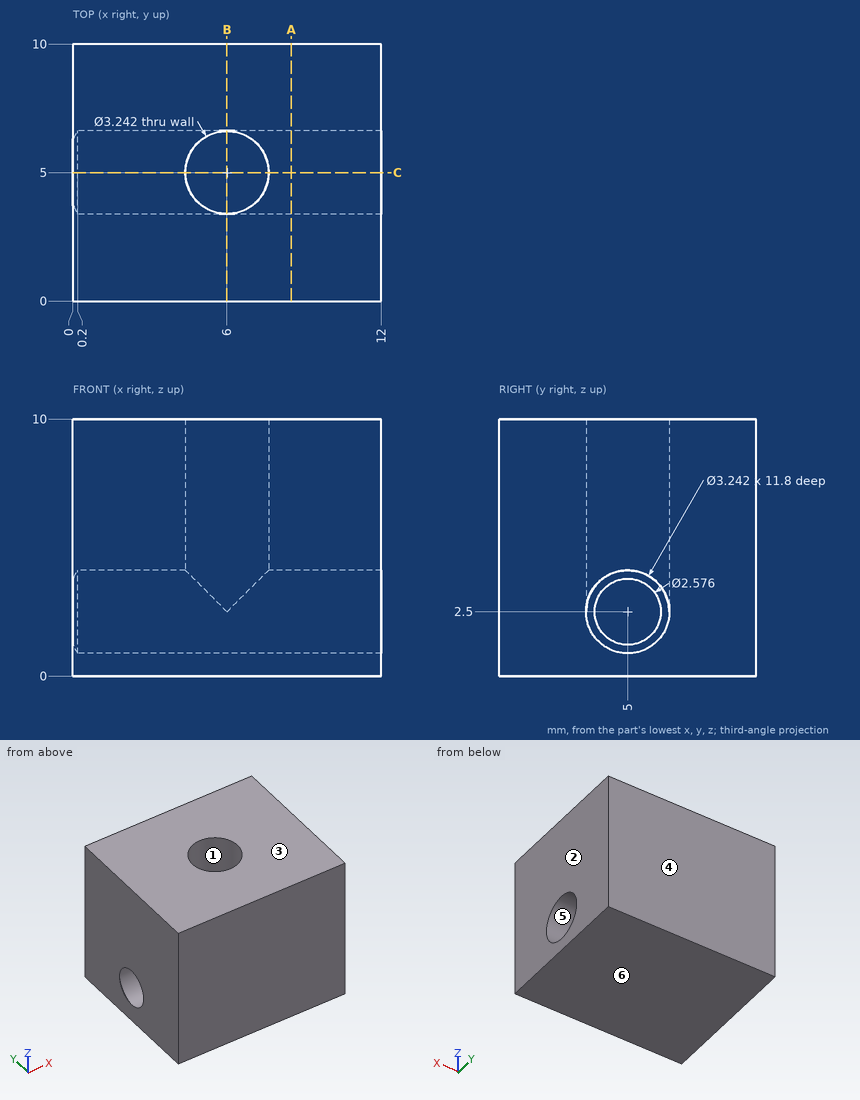
Here's the drawing with two shaded views (mm, measured from the low corner). I have some questions. A direction names the side the tool comes from. Round coordinates to 2 decimals unless told otherwise and drop trailing zeros. Write each loop counter-clockwise with the first axis right and the second up, starting at its lowest first coordinate (ties: lowest second). Pieces come first, ordered by that corner, then holes. Notation, with made-up numbers: M 22.5,75 L 67.5,75 A23 ccw 67.5,113 Z; hole C 42.25,-14 d7. An arc over 180 degrees is marked long. Write each question's results on one line, items separated by ' | '. Start each with the question number.
1. Imagine slicing it at B-B on x = 6. List the corners of the cut face in (y, z) for me.
2. Thinking about a two-plate mould opening in Z: for the marked faces 3, 4, 5 and 6, which applies, +Z half, -Z half, draft (parallel to the pull), parting line (faces both ways), or undercut?
3. I need wall thicknesses on L1, parallel to Y at x = 4.5, z = 2.5; L2, parallel to Z at x = 11, y = 4 (1 decimal); L3, parallel to Y at x = 6, z = 1.5 (1 decimal). Which ranges of each line are inside material? Lowest first, please. Write a range as from..to.
4. Imagine slicing it at C-C on y = 5. List the corners of the cut face in (x, z) for me.
5. Imagine slicing it at A-A on x = 8.5. List the corners of the cut face in (y, z) for me.
6. On a 3-axis mill with a long thin cutter (end or side, diameter ignored), from which of +Z, -Z, +X, -X, +Y, -Y can I reach the whole of each face in a straight line? I mean the marked faces 1 and 2. Say none if no direction works.
Result sheet:
1) outline: M 0,0 L 10,0 L 10,10 L 6.62,10 L 6.62,2.5 A1.62 cw 3.38,2.5 L 3.38,10 L 0,10 Z
2) face 3: +Z half | face 4: draft | face 5: undercut | face 6: -Z half
3) L1: y = 0..3.38, 6.62..10 | L2: z = 0..1.2, 3.8..10 | L3: y = 0..3.7, 6.3..10
4) outline: M 0,0 L 12,0 L 12,0.88 L 0.2,0.88 L 0,1.21 Z; M 0,3.79 L 0.2,4.12 L 4.38,4.12 L 4.38,10 L 0,10 Z; M 7.62,4.12 L 12,4.12 L 12,10 L 7.62,10 Z
5) outline: M 0,0 L 10,0 L 10,10 L 0,10 Z; hole C 5,2.5 d3.24
6) face 1: +Z | face 2: +Z, -Z, +X, +Y, -Y
